Here's the drawing with two shaded views (mm, measured from the low corner). I have some questions. Coordinates: 2 decimals unless noted, no trailing zeros. Write each loop counter-clockwise with the first axis right and the second up, starting at its lowest first coordinate (ties: lowest second). Pieces come first, ordered by that corner, then holes. Notation, with made-up numbers: (15.5, 82.25) -> (56.5, 82.25) arc R8 ccw to (56.5, 90.25) -> close; hole circle Ø3 at (15.25, 24.5). An arc over 180 degrees is marked (long way). Use one line per item in the form item = value.
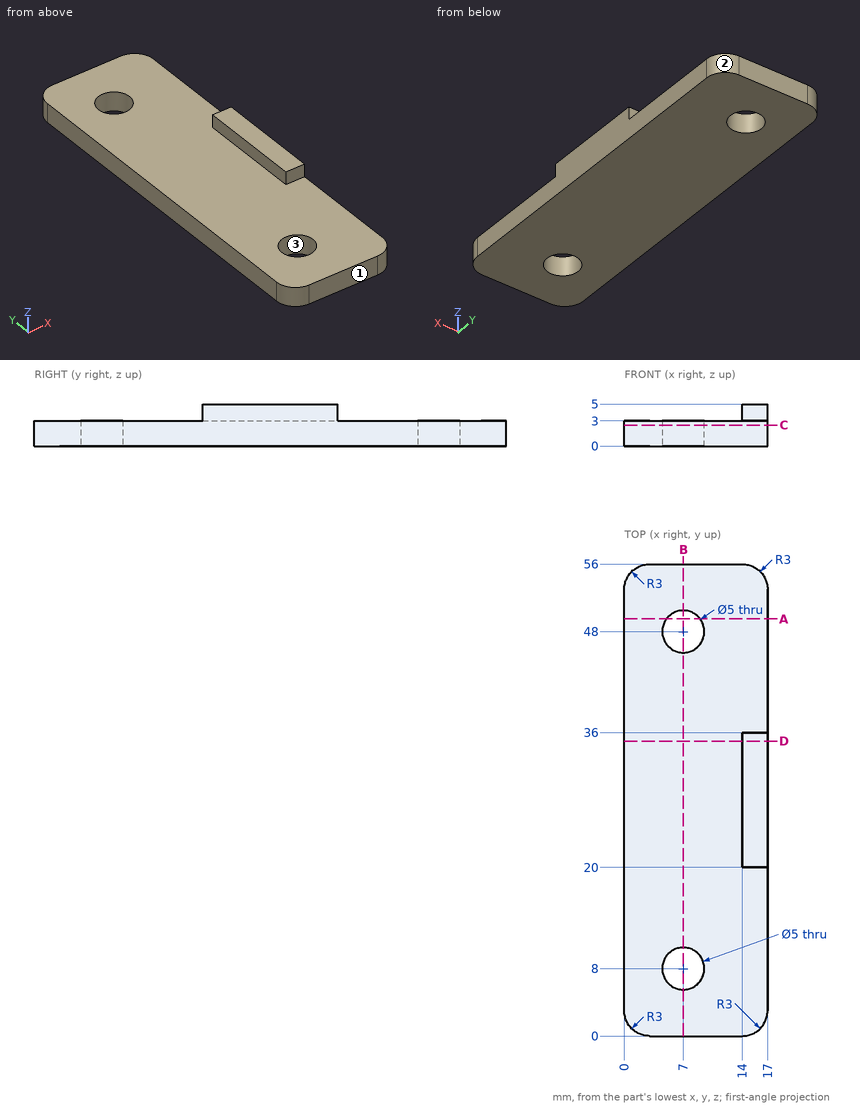
Q1. If I drill on line 1 (Y direction, x = 7, z = 1.8); line 2 (Y direction, x = 14.25, z = 3.55); line 3 (Z direction, x = 6.75, y = 4.5), over which ranges is the centre line in solid material (lowest first)? Write a range as from..to.
Return value:
line_1 = 0..5.5, 10.5..45.5, 50.5..56
line_2 = 20..36
line_3 = 0..3
Q2. Suppose I cut it at D-D (y = 35). Write out the boundary of the cut face in (x, z).
Return value:
outline = (0, 0) -> (17, 0) -> (17, 5) -> (14, 5) -> (14, 3) -> (0, 3) -> close
Q3. Suppose I cut it at C-C (z = 2.5). Write out the boundary of the cut face in (x, y).
Return value:
outline = (0, 3) arc R3 ccw to (3, 0) -> (14, 0) arc R3 ccw to (17, 3) -> (17, 53) arc R3 ccw to (14, 56) -> (3, 56) arc R3 ccw to (0, 53) -> close; hole circle Ø5 at (7, 8); hole circle Ø5 at (7, 48)
Q4. Suppose I cut it at A-A (y = 49.5). Write out the boundary of the cut face in (x, z).
Return value:
outline = (0, 0) -> (5, 0) -> (5, 3) -> (0, 3) -> close; (9, 0) -> (17, 0) -> (17, 3) -> (9, 3) -> close
Q5. Thinking about a two-plate mould opening in X: for the marked faces 1, 2 and 3, which applies, released by +X, released by -X, zero draft, split by the parting line, or undercut?
Return value:
face_1 = zero draft
face_2 = released by +X
face_3 = undercut
Q6. Suppose I cut it at B-B (x = 7). Write out the boundary of the cut face in (y, z), then the cut area to 3 significant figures.
Return value:
outline = (0, 0) -> (5.5, 0) -> (5.5, 3) -> (0, 3) -> close; (10.5, 0) -> (45.5, 0) -> (45.5, 3) -> (10.5, 3) -> close; (50.5, 0) -> (56, 0) -> (56, 3) -> (50.5, 3) -> close
area = 138 mm2
Q7. Will these pins go through, and if not, where does the flat tip stop? pin 1 (3 mm diameter, centred on x = 9, z = 1, fed in from -Y); pin 2 (1 mm diameter, centred on y = 31, z = 4, fed in from -X); pin 3 (3 mm diameter, centred on x = 7, y = 48, fed in from +Z); pin 4 (1.6 mm diameter, centred on x = 15, z = 4, fed in from -Y).
Return value:
pin_1 = 0
pin_2 = 14
pin_3 = through
pin_4 = 20
